Read the model definition and answer for the solid it produces. Units are mm, in the model's axes. Face numbers are marked on the shaded views. A direction names the side the tool comes from. Coordinates: 2 decimals unless noted, no trailing zeros. Loops run counter-clockwise (first coordinate to the right, second up) from the corner with the lowest first, then second, coordinate; pieces in that order, holes last.
Q1. Section B-B (y = -11) is taken. Give the vertices of the cut face in (x, z), then the cut area to 3 significant figures.
Q2. Flat-ended cylindrical pins translate along their axes: P1, Ø3, axis at x = 1.5, y = -18.5, coming from the +Z side; P2, Ø1, axis at x = -1.5, y = -16, coming from the -Z side; P3, Ø1.5, axis at y = -11.5, z = 2.5, coming from the -X side; P4, Ø2, axis at x = 0.5, z = -0.5, coming from the -Y side. Find the tip coordinate at first contact, or state that the pin passes through.
Q3. Section A-A (y = -25.5) is taken. Give the vertices of the cut face in (x, z).
Q4. Which of the six approach directions +Z, -Z, +X, -X, +Y, -Y give full straight-line access (tool end or side, diameter ignored) to the marked faces 1 and 2?
Q5. Straight lines are drawn through the part: line 1 (Z direction, x = -2, y = -21.5); line 2 (Z direction, x = 0.5, y = -9.75); line 3 (Y direction, x = -1.5, z = 2.75). For each, find the intervals that lie inside material, in ascending order.
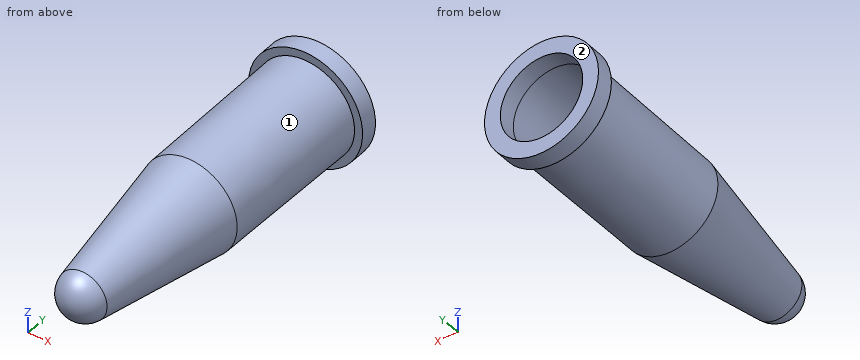
from build123d import *

# Parameters (mm, degrees)
BOSS_EXTRUDE4_DEPTH = 2.000034
SCALE1_SCALE        = 0.510872955


with BuildPart() as part:
    # Sketch1 → Revolve25 (revolve)
    with BuildSketch(Plane.XY):
        with BuildLine():
            Line((-4.682614804, -1.992146118), (-4.7, 0))
            Line((-4.7, 0), (-6.5, 0))
            Line((-6.5, 0), (-6.5, -2))
            Line((-6.5, -2), (-5.582580535, -2))
            Line((-5.582580535, -2), (-5.425496915, -20))
            Line((-5.425496915, -20), (-2.794168337, -36.613554791))
            ThreePointArc((-2.794168337, -36.613554791), (-1.837287228, -38.322188957), (0, -39))
            Line((0, -39), (0, -38.1))
            ThreePointArc((0, -38.1), (-1.252783984, -37.637823588), (-1.905248831, -36.472763773))
            Line((-1.905248831, -36.472763773), (-4.526114828, -19.925267112))
            Line((-4.526114828, -19.925267112), (-4.682614804, -1.992146118))
        make_face()
    revolve(axis=Axis((0, 0, 0), (0, -1, 0)))


with BuildPart() as body_2:
    # Sketch1<10> → Revolve31 (revolve)
    with BuildSketch(Plane.XY):
        Polygon((22, 2.999966443), (22, 1.999966443), (26, 1.999966443), (26, -2.000033557), (28.5, -2.000033557), (28.5, 0), (26.7, 0), (26.569018636, 2.999966443), align=None)
    revolve(axis=Axis((22, 17.95552364, 0), (0, -1, 0)))

    # Sketch2 → Boss-Extrude4 (add)
    with BuildSketch(Plane(origin=(0, -2.000033557, 0), x_dir=(-1, 0, 0), z_dir=(0, -1, 0))):
        with BuildLine():
            Line((-22, 4), (-22, 6.5))
            add(Edge.make_bspline(
                [(-22, 6.5), (-30.5, 6.5), (-30.5, 0), (-30.5, -6.5), (-22, -6.5)],
                knots=[1.570796327, 1.570796327, 1.570796327, 3.141592654, 3.141592654, 4.71238898, 4.71238898, 4.71238898], degree=2, weights=[1, 0.707106781, 1, 0.707106781, 1]))
            Line((-22, -6.5), (-22, -4))
            ThreePointArc((-22, -4), (-26, 0), (-22, 4))
        make_face()
    extrude(amount=-BOSS_EXTRUDE4_DEPTH)


with BuildPart() as part_1:
    # Scale1: scaled about (0, -15.998689943, 0)
    add(part.part.scale(SCALE1_SCALE).moved(Location((0, -7.825391937, 0))))


solid = part_1.part
Numbers:
1. outline: circle Ø5.67 at (0, 0); hole circle Ø4.75 at (0, 0)
1. area: 7.52 mm2
2. P1: stops at z = 2.77
2. P2: stops at z = -2.6
2. P3: stops at x = -2.22
2. P4: stops at y = -27.75
3. outline: circle Ø3.18 at (0, 0); hole circle Ø2.25 at (0, 0)
4. face 1: -Y
4. face 2: +Z, -Z, +X, -X, +Y
5. line 1: z = -0.97 to 0.97
5. line 2: z = -2.8 to -2.33, 2.33 to 2.8
5. line 3: y = -8.85 to -7.83
